Read the model definition and answer for the solid it produces. Units are mm, in the model's axes. Face numbers are marked on the shaded views. A direction names the side the tool comes from. Coordinates: 2 decimals unless noted, no trailing zeros. Write each loop counter-clockwise with the first axis right and the second up, starting at its lowest first coordinate (ties: lowest second). Pieces come first, ordered by that corner, then holes.
(1) Section B-B on z = -2.5 is taken. Write down the section's boundary in (x, y).
(2) Given pin 1 (5 mm diameter, centred on x = -3.5, y = -2, fed in from -Z); pin 2 (1 mm diameter, centred on x = -2, y = 7, fed in from +Z); pin 3 (3 mm diameter, centred on y = -2, z = 2.5, fed in from -X), each flat-ended and moving along its own axis, determine where each tip first touches the part or whether it passes through.
(3) Section D-D on z = -5 is taken. Write down the section's boundary in (x, y).
(4) Find the intervals of material crossed by probe 1 along X at (y, z) = (6.5, 0.75); probe 2 along X at (y, z) = (-6, -2.5); probe 3 along Z at (x, y) = (-0.25, 9), in increasing order.
(5) The mould has two halves that part along Z. Classify the marked faces 1, 2 and 3: +Z half, -Z half, draft (parallel to the pull), parting line (faces both ways), or undercut.
(6) Section C-C on y = -8 is taken. Write down the section's boundary in (x, z), then the cut area to 3 significant figures.
(7) Which of the six approach directions +Z, -Z, +X, -X, +Y, -Y give full straight-line access (tool end or side, diameter ignored) to the marked faces 4 and 5?
(8) Section A-A on x = -0.5 is taken. Write down the section's boundary in (y, z).
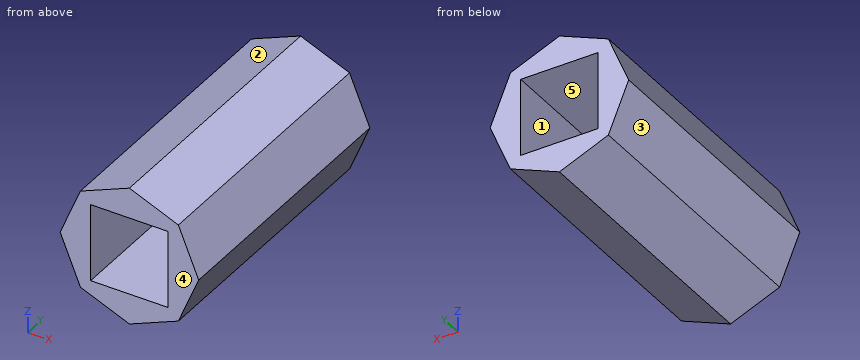
from build123d import *

# Parameters (mm, degrees)
SKETCH1_W           = 6.731
SKETCH1_H           = 6.731
BOSS_EXTRUDE1_DEPTH = 11.90625


with BuildPart() as part:
    # Sketch1 → Boss-Extrude1 (new, symmetric)
    with BuildSketch(Plane(origin=(0, 0, 0), x_dir=(1, 0, 0), z_dir=(0, 1, 0))):
        Polygon((6.014041663, 0), (4.252569642, 4.252569642), (0, 6.014041663), (-4.252569642, 4.252569642), (-6.014041663, 0), (-4.252569642, -4.252569642), (0, -6.014041663), (4.252569642, -4.252569642), align=None)
        Rectangle(SKETCH1_W, SKETCH1_H, mode=Mode.SUBTRACT)
    extrude(amount=BOSS_EXTRUDE1_DEPTH, both=True)


solid = part.part
Response:
1. outline: (-4.98, -11.91) - (-3.37, -11.91) - (-3.37, 11.91) - (-4.98, 11.91) - close; (3.37, -11.91) - (4.98, -11.91) - (4.98, 11.91) - (3.37, 11.91) - close
2. pin 1: stops at z = -5.6
2. pin 2: stops at z = 5.39
2. pin 3: stops at x = -5.6
3. outline: (-2.45, -11.91) - (2.45, -11.91) - (2.45, 11.91) - (-2.45, 11.91) - close
4. probe 1: x = -5.7 to -3.37, 3.37 to 5.7
4. probe 2: x = -4.98 to -3.37, 3.37 to 4.98
4. probe 3: z = -5.91 to -3.37, 3.37 to 5.91
5. face 1: undercut
5. face 2: +Z half
5. face 3: -Z half
6. outline: (-6.01, 0) - (-4.25, -4.25) - (0, -6.01) - (4.25, -4.25) - (6.01, 0) - (4.25, 4.25) - (0, 6.01) - (-4.25, 4.25) - close; hole (-3.37, -3.37) - (3.37, -3.37) - (3.37, 3.37) - (-3.37, 3.37) - close
6. area: 57.0 mm2
7. face 4: +Z, -Z, +X, -X, -Y
7. face 5: +Y, -Y
8. outline: (-11.91, -5.81) - (11.91, -5.81) - (11.91, -3.37) - (-11.91, -3.37) - close; (-11.91, 3.37) - (11.91, 3.37) - (11.91, 5.81) - (-11.91, 5.81) - close
